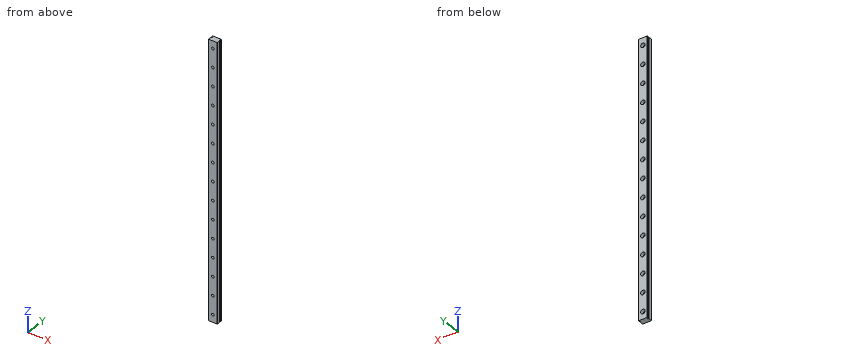
from build123d import *

# Parameters (mm, degrees)
EXTRUDE_1_DEPTH        = 370
SKETCH_2_R             = 3
SKETCH_2_R_2           = 1.75
CUT_EXTRUDE_1_DEPTH    = 4.5
SKETCH_2_2_R           = 1.75
CUT_EXTRUDE_2_DEPTH    = 9
PATTERN_LINEAR_1_COUNT = 16
PATTERN_LINEAR_1_PITCH = 25


with BuildPart() as part:
    # Эскиз1 → Бобышка-Вытянуть1 (new body)
    with BuildSketch(Plane.XY):
        with BuildLine():
            Line((-6, 3.7), (-5.7, 4))
            Line((-5.7, 4), (5.7, 4))
            Line((5.7, 4), (6, 3.7))
            Line((6, 3.7), (6, 2.451013544))
            ThreePointArc((6, 2.451013544), (5.597935912, 2.202976267), (5.354599002, 1.798050138))
            Line((5.354599002, 1.798050138), (4.643514056, 1.798050138))
            Line((4.643514056, 1.798050138), (4.643514056, 1.201949862))
            Line((4.643514056, 1.201949862), (5.354599002, 1.201949862))
            ThreePointArc((5.354599002, 1.201949862), (5.597935912, 0.797023733), (6, 0.548986456))
            Line((6, 0.548986456), (6, -3.7))
            Line((6, -3.7), (5.7, -4))
            Line((5.7, -4), (-5.7, -4))
            Line((-5.7, -4), (-6, -3.7))
            Line((-6, -3.7), (-6, 0.548986456))
            ThreePointArc((-6, 0.548986456), (-5.597935912, 0.797023733), (-5.354599002, 1.201949862))
            Line((-5.354599002, 1.201949862), (-4.643514056, 1.201949862))
            Line((-4.643514056, 1.201949862), (-4.643514056, 1.798050138))
            Line((-4.643514056, 1.798050138), (-5.354599002, 1.798050138))
            ThreePointArc((-5.354599002, 1.798050138), (-5.597935912, 2.202976267), (-6, 2.451013544))
            Line((-6, 2.451013544), (-6, 3.7))
        make_face()
    extrude(amount=EXTRUDE_1_DEPTH)

    # Эскиз2 → Вырез-Вытянуть1 (cut)
    with BuildSketch(Plane(origin=(0, 4, 0), x_dir=(1, 0, 0), z_dir=(0, 1, 0))):
        with Locations((0, -10)):
            Circle(SKETCH_2_R)
        with Locations((0, -10)):
            Circle(SKETCH_2_R_2, mode=Mode.SUBTRACT)
    cut_extrude_1 = extrude(amount=-CUT_EXTRUDE_1_DEPTH, mode=Mode.SUBTRACT)

    # Эскиз2<2> → Вырез-Вытянуть2 (cut, through all)
    with BuildSketch(Plane(origin=(0, 4, 0), x_dir=(1, 0, 0), z_dir=(0, 1, 0))):
        with Locations((0, -10)):
            Circle(SKETCH_2_2_R)
    cut_extrude_2 = extrude(amount=-CUT_EXTRUDE_2_DEPTH, mode=Mode.SUBTRACT)

    # Линейный массив1: Вырез-Вытянуть1, Вырез-Вытянуть2 ×16
    with Locations(*[(0, 0, i * PATTERN_LINEAR_1_PITCH) for i in range(1, PATTERN_LINEAR_1_COUNT)]):
        add(cut_extrude_1, mode=Mode.SUBTRACT)
        add(cut_extrude_2, mode=Mode.SUBTRACT)


solid = part.part
Input: part model. Units: mm. Frame: model coordinates. Round coordinates to 2 decimals unless told otherwise and drop trailing zeros. Order: outer loops, then holes, each group sorted by start corner. A loop starts at its lowest first (then second) coordinate and runs counter-clockwise, first axis right, second up.
1. Cut plane A-A, the plane z = 321. Output: boundary loops of the cut face in (x, y), then the cut area to 3 significant figures.
The answers:
outline: (-6, -3.7) - (-5.7, -4) - (5.7, -4) - (6, -3.7) - (6, 0.55) arc R1 cw to (5.35, 1.2) - (4.64, 1.2) - (4.64, 1.8) - (5.35, 1.8) arc R1 cw to (6, 2.45) - (6, 3.7) - (5.7, 4) - (-5.7, 4) - (-6, 3.7) - (-6, 2.45) arc R1 cw to (-5.35, 1.8) - (-4.64, 1.8) - (-4.64, 1.2) - (-5.35, 1.2) arc R1 cw to (-6, 0.55) - close
area: 93.1 mm2
2. Pin query (flat end, axial travel): P1, Ø5.5, axis at x = 0, z = 360, coming from the +Y side; P2, Ø3, axis at x = 0, z = 160, coming from the -Y side. Return the tip coordinate at first contact, or that it passes through.
The answers:
P1: stops at y = -0.5
P2: passes through
3. Material intervals for line 1 (X direction, y = -1.9, z = 210); line 2 (X direction, y = 1.5, z = 130); line 3 (Y direction, x = -2, z = 209.5), sorted ascending.
The answers:
line 1: x = -6 to -1.75, 1.75 to 6
line 2: x = -4.64 to 4.64
line 3: y = -4 to -0.5
